from build123d import *

# Parameters (mm, degrees)
BOSS_EXTRUDE1_DEPTH = 3.175
SKETCH2_R           = 1.5875
CUT_EXTRUDE1_DEPTH  = 4.175
BOSS_EXTRUDE2_DEPTH = 3.175


with BuildPart() as part:
    # Sketch1 → Boss-Extrude1 (new body)
    with BuildSketch(Plane(origin=(0, 0, 0), x_dir=(1, 0, 0), z_dir=(0, 1, 0))):
        Polygon((0, 50.8), (0, 0), (88.9, 0), (88.9, 38.1), (38.1, 38.1), (38.1, 50.8), align=None)
    extrude(amount=BOSS_EXTRUDE1_DEPTH)

    # Sketch2 → Cut-Extrude1 (cut, through all)
    with BuildSketch(Plane(origin=(0, 3.175, 0), x_dir=(1, 0, 0), z_dir=(0, 1, 0))):
        with Locations((6.35, 44.45)):
            Circle(SKETCH2_R)
        with Locations((31.75, 44.45)):
            Circle(SKETCH2_R)
        with Locations((31.75, 31.75)):
            Circle(SKETCH2_R)
        with Locations((6.35, 31.75)):
            Circle(SKETCH2_R)
        with Locations((6.35, 6.35)):
            Circle(SKETCH2_R)
        with Locations((31.75, 6.35)):
            Circle(SKETCH2_R)
        with Locations((82.55, 6.35)):
            Circle(SKETCH2_R)
        with Locations((82.55, 31.75)):
            Circle(SKETCH2_R)
        with Locations((57.15, 31.75)):
            Circle(SKETCH2_R)
        with Locations((57.15, 6.35)):
            Circle(SKETCH2_R)
        with Locations((44.45, 6.35)):
            Circle(SKETCH2_R)
        with Locations((44.45, 31.75)):
            Circle(SKETCH2_R)
    extrude(amount=-CUT_EXTRUDE1_DEPTH, mode=Mode.SUBTRACT)

    # Sketch3 → Boss-Extrude2 (add)
    with BuildSketch(Plane(origin=(0, 3.175, 0), x_dir=(1, 0, 0), z_dir=(0, 1, 0))):
        Polygon((0, 101.6), (38.1, 101.6), (139.7, 38.1), (139.7, 0), (88.9, 0), (88.9, 38.1), (38.1, 38.1), (38.1, 50.8), (0, 50.8), align=None)
    extrude(amount=-BOSS_EXTRUDE2_DEPTH)


solid = part.part
Model file for the job. Use its own axes, mm. Give positions to 0.01 mm unless a question says otherwise; leave off trailing zeros. Loops run counter-clockwise (first coordinate to the right, second up) from the corner with the lowest first, then second, coordinate; pieces in that order, holes last. Notation, with made-up numbers: (13, 50.25) -> (42, 50.25) arc R36 ccw to (42, 84.25) -> close; hole circle Ø2 at (50, 30). An arc over 180 degrees is marked (long way). Use a Markdown table: item, result. Add a question column.
(1) Slice it at C-C on y = 2.3. Give the number of separate pieces and of enclosed holes in the cut face, and give its area (3 significant figures).
(2) Slice it at D-D on x = 6.35. List the corners of the cut face in (y, z) (1 decimal).
(3) Mould opens along Z. For faces 1 (the flat face through (71, 2, 0)), 2 (the flat face through (55, 0, -40)), 3 (the cylindrical face through (32.48, 1.61, -43.04)) say: +Z half, -Z half, draft (parallel to the pull), parting line (faces both ways), or undercut.
(4) Slice it at B-B on z = -44.45. List the corners of the cut face in (x, y) (1 decimal), and give its area (3 significant figures).
(5) Wall check: line 1 along X through (y, z) = (2.3, -6.35); line 2 along Z through (x, y) = (6.35, 1.65); line 3 along Z through (x, y) = (44.45, 2.3). Give the ranges that are in metal, low to high.
(6) Slice it at A-A on z = -6.35. List the corners of the cut face in (x, y) (1 decimal), and give its area (3 significant figures).
Filled sheet:
| question | item | result |
|---|---|---|
| 1 | separate pieces | 1 |
| 1 | enclosed holes | 12 |
| 1 | area | 10,900 mm2 |
| 2 | outline | (0, -101.6) -> (3.2, -101.6) -> (3.2, -46) -> (0, -46) -> close; (0, -42.9) -> (3.2, -42.9) -> (3.2, -33.3) -> (0, -33.3) -> close; (0, -30.2) -> (3.2, -30.2) -> (3.2, -7.9) -> (0, -7.9) -> close; (0, -4.8) -> (3.2, -4.8) -> (3.2, 0) -> (0, 0) -> close |
| 3 | face 1 | +Z half |
| 3 | face 2 | draft |
| 3 | face 3 | undercut |
| 4 | outline | (0, 0) -> (4.8, 0) -> (4.8, 3.2) -> (0, 3.2) -> close; (7.9, 0) -> (30.2, 0) -> (30.2, 3.2) -> (7.9, 3.2) -> close; (33.3, 0) -> (129.5, 0) -> (129.5, 3.2) -> (33.3, 3.2) -> close |
| 4 | area | 391 mm2 |
| 5 | line 1 | 0 to 4.76, 7.94 to 30.16, 33.34 to 42.86, 46.04 to 55.56, 58.74 to 80.96, 84.14 to 139.7 |
| 5 | line 2 | -101.6 to -46.04, -42.86 to -33.34, -30.16 to -7.94, -4.76 to 0 |
| 5 | line 3 | -97.63 to -33.34, -30.16 to -7.94, -4.76 to 0 |
| 6 | outline | (0, 0) -> (4.8, 0) -> (4.8, 3.2) -> (0, 3.2) -> close; (7.9, 0) -> (30.2, 0) -> (30.2, 3.2) -> (7.9, 3.2) -> close; (33.3, 0) -> (42.9, 0) -> (42.9, 3.2) -> (33.3, 3.2) -> close; (46, 0) -> (55.6, 0) -> (55.6, 3.2) -> (46, 3.2) -> close; (58.7, 0) -> (81, 0) -> (81, 3.2) -> (58.7, 3.2) -> close; (84.1, 0) -> (139.7, 0) -> (139.7, 3.2) -> (84.1, 3.2) -> close |
| 6 | area | 393 mm2 |
